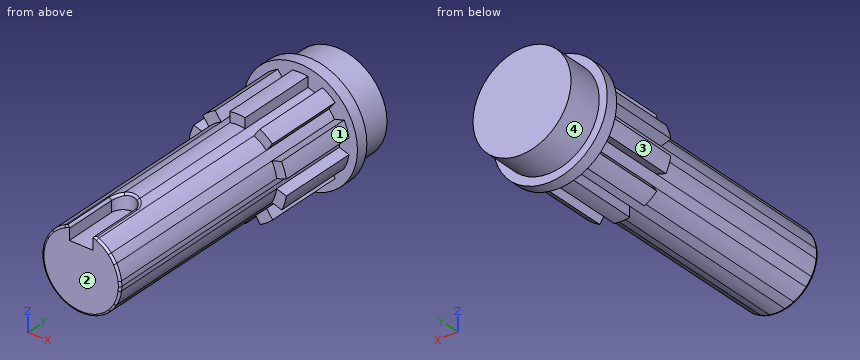
from build123d import *

# Parameters (mm, degrees)
F1_R     = 14.5
F1_R_2   = 12.45
F2_DEPTH = 3
F3_DEPTH = 12
F4_DEPTH = 20
F5_DEPTH = 70
F8_DEPTH = 25
F9_R     = 0.5


with BuildPart() as f2:
    # F1 (on Front) → F2 (new body)
    with BuildSketch(Plane.XZ):
        Circle(F1_R)
        Circle(F1_R_2, mode=Mode.SUBTRACT)
    extrude(amount=-F2_DEPTH)

    # F1 (on Front) → F3 (join)
    with BuildSketch(Plane.XZ):
        Circle(F1_R_2)
    extrude(amount=-F3_DEPTH)

    # F0 (on Front) → F4 (join)
    with BuildSketch(Plane.XZ):
        with BuildLine():
            ThreePointArc((-7.324554284, 6.7344936366), (-5.8782605878, 8.0279855793), (-4.2084272228, 9.0161876816))
            Line((-4.2084272228, 9.0161876816), (-5.7294038305, 11.1096323858))
            ThreePointArc((-5.7294038305, 11.1096323858), (-7.3861439392, 10.0843878203), (-8.8634461682, 8.8141546403))
            Line((-8.8634461682, 8.8141546403), (-7.324554284, 6.7344936366))
        make_face()
        with BuildLine():
            ThreePointArc((-1.9672528507, 9.7535847882), (-0.0368811837, 9.9499316469), (1.8948930083, 9.7679005158))
            Line((1.8948930083, 9.7679005158), (1.8948930083, 12.3555404773))
            ThreePointArc((1.8948930083, 12.3555404773), (-0.0480615306, 12.4999076032), (-1.9898484698, 12.3406038372))
            Line((-1.9898484698, 12.3406038372), (-1.9672528507, 9.7535847882))
        make_face()
        with BuildLine():
            ThreePointArc((4.141472307, 9.047138063), (5.818585579, 8.0713420111), (7.2744285153, 6.7886073517))
            Line((7.2744285153, 6.7886073517), (8.7954051229, 8.8820520559))
            ThreePointArc((8.7954051229, 8.8820520559), (7.3083787492, 10.140887538), (5.6438037116, 11.15336181))
            Line((5.6438037116, 11.15336181), (4.141472307, 9.047138063))
        make_face()
        with BuildLine():
            ThreePointArc((8.668295807, 4.8849920985), (9.4515504169, 3.1097740619), (9.8753795782, 1.2162969155))
            Line((9.8753795782, 1.2162969155), (12.3363714254, 2.015921639))
            ThreePointArc((12.3363714254, 2.015921639), (11.8732667494, 3.9083931094), (11.121714701, 5.7059146602))
            Line((11.121714701, 5.7059146602), (8.668295807, 4.8849920985))
        make_face()
        with BuildLine():
            Line((12.3515086878, -1.9209979529), (9.8841249332, -1.1430548127))
            ThreePointArc((9.8841249332, -1.1430548127), (9.474344242, -3.0396218816), (8.704271294, -4.820597602))
            Line((8.704271294, -4.820597602), (11.1652631412, -5.6202223254))
            ThreePointArc((11.1652631412, -5.6202223254), (11.9029704089, -3.8169746457), (12.3515086878, -1.9209979529))
        make_face()
        with BuildLine():
            Line((8.8634461682, -8.8141546403), (7.324554284, -6.7344936366))
            ThreePointArc((7.324554284, -6.7344936366), (5.8782605878, -8.0279855793), (4.2084272228, -9.0161876816))
            Line((4.2084272228, -9.0161876816), (5.7294038305, -11.1096323858))
            ThreePointArc((5.7294038305, -11.1096323858), (7.3861439392, -10.0843878203), (8.8634461682, -8.8141546403))
        make_face()
        with BuildLine():
            Line((1.9898484698, -12.3406038372), (1.9672528507, -9.7535847882))
            ThreePointArc((1.9672528507, -9.7535847882), (0.0368811837, -9.9499316469), (-1.8948930083, -9.7679005158))
            Line((-1.8948930083, -9.7679005158), (-1.8948930083, -12.3555404773))
            ThreePointArc((-1.8948930083, -12.3555404773), (0.0480615306, -12.4999076032), (1.9898484698, -12.3406038372))
        make_face()
        with BuildLine():
            Line((-5.6438037116, -11.15336181), (-4.141472307, -9.047138063))
            ThreePointArc((-4.141472307, -9.047138063), (-5.818585579, -8.0713420111), (-7.2744285153, -6.7886073517))
            Line((-7.2744285153, -6.7886073517), (-8.7954051229, -8.8820520559))
            ThreePointArc((-8.7954051229, -8.8820520559), (-7.3083787492, -10.140887538), (-5.6438037116, -11.15336181))
        make_face()
        with BuildLine():
            Line((-11.121714701, -5.7059146602), (-8.668295807, -4.8849920985))
            ThreePointArc((-8.668295807, -4.8849920985), (-9.4515504169, -3.1097740619), (-9.8753795782, -1.2162969155))
            Line((-9.8753795782, -1.2162969155), (-12.3363714254, -2.015921639))
            ThreePointArc((-12.3363714254, -2.015921639), (-11.8732667494, -3.9083931094), (-11.121714701, -5.7059146602))
        make_face()
        with BuildLine():
            ThreePointArc((-9.8841249332, 1.1430548127), (-9.474344242, 3.0396218816), (-8.704271294, 4.820597602))
            Line((-8.704271294, 4.820597602), (-11.1652631412, 5.6202223254))
            ThreePointArc((-11.1652631412, 5.6202223254), (-11.9029704089, 3.8169746457), (-12.3515086878, 1.9209979529))
            Line((-12.3515086878, 1.9209979529), (-9.8841249332, 1.1430548127))
        make_face()
    extrude(amount=F4_DEPTH)

    # F0 (on Front) → F5 (join)
    with BuildSketch(Plane.XZ):
        with BuildLine():
            ThreePointArc((9.8841249332, -1.1430548127), (9.9335175815, -0.5724757264), (9.95, 0))
            ThreePointArc((9.95, 0), (9.9313273736, 0.6092918829), (9.8753795782, 1.2162969155))
            ThreePointArc((9.8753795782, 1.2162969155), (9.4515504169, 3.1097740619), (8.668295807, 4.8849920985))
            ThreePointArc((8.668295807, 4.8849920985), (8.0279855793, 5.8782605878), (7.2744285153, 6.7886073517))
            ThreePointArc((7.2744285153, 6.7886073517), (5.818585579, 8.0713420111), (4.141472307, 9.047138063))
            ThreePointArc((4.141472307, 9.047138063), (3.0396218816, 9.474344242), (1.8948930083, 9.7679005158))
            ThreePointArc((1.8948930083, 9.7679005158), (-0.0368811837, 9.9499316469), (-1.9672528507, 9.7535847882))
            ThreePointArc((-1.9672528507, 9.7535847882), (-3.1097740619, 9.4515504169), (-4.2084272228, 9.0161876816))
            ThreePointArc((-4.2084272228, 9.0161876816), (-5.8782605878, 8.0279855793), (-7.324554284, 6.7344936366))
            ThreePointArc((-7.324554284, 6.7344936366), (-8.0713420111, 5.818585579), (-8.704271294, 4.820597602))
            ThreePointArc((-8.704271294, 4.820597602), (-9.474344242, 3.0396218816), (-9.8841249332, 1.1430548127))
            ThreePointArc((-9.8841249332, 1.1430548127), (-9.9499316469, -0.0368811837), (-9.8753795782, -1.2162969155))
            ThreePointArc((-9.8753795782, -1.2162969155), (-9.4515504169, -3.1097740619), (-8.668295807, -4.8849920985))
            ThreePointArc((-8.668295807, -4.8849920985), (-8.0279855793, -5.8782605878), (-7.2744285153, -6.7886073517))
            ThreePointArc((-7.2744285153, -6.7886073517), (-5.818585579, -8.0713420111), (-4.141472307, -9.047138063))
            ThreePointArc((-4.141472307, -9.047138063), (-3.0396218816, -9.474344242), (-1.8948930083, -9.7679005158))
            ThreePointArc((-1.8948930083, -9.7679005158), (0.0368811837, -9.9499316469), (1.9672528507, -9.7535847882))
            ThreePointArc((1.9672528507, -9.7535847882), (3.1097740619, -9.4515504169), (4.2084272228, -9.0161876816))
            ThreePointArc((4.2084272228, -9.0161876816), (5.8782605878, -8.0279855793), (7.324554284, -6.7344936366))
            ThreePointArc((7.324554284, -6.7344936366), (8.0713420111, -5.818585579), (8.704271294, -4.820597602))
            ThreePointArc((8.704271294, -4.820597602), (9.474344242, -3.0396218816), (9.8841249332, -1.1430548127))
        make_face()
    extrude(amount=F5_DEPTH)

    # F7 (on offset) → F8 (cut)
    with BuildSketch(Plane.XY.offset(6)):
        with BuildLine():
            Line((-3, -74.6025964618), (0, -74.6025964618))
            Line((0, -74.6025964618), (3, -74.6025964618))
            Line((3, -74.6025964618), (3, -56.6025964618))
            ThreePointArc((3, -56.6025964618), (0, -53.6025964618), (-3, -56.6025964618))
            Line((-3, -56.6025964618), (-3, -74.6025964618))
        make_face()
    extrude(amount=F8_DEPTH, mode=Mode.SUBTRACT)

    # F9
    f9_edges = [f2.edges().sort_by_distance(p)[0] for p in [
        (-3, -63.301298, 9.486965),
        (0, -53.602596, 9.95),
        (3, -63.301298, 9.486965),
        (-5.377611, -70, -8.371607),
        (7.65146, -70, 6.360634),
    ]]
    fillet(f9_edges, radius=F9_R)


solid = f2.part
Geometry check sheet. Reference: the model listing, model coordinates, mm. Face numbers are marked on the shaded views. A direction names the side the tool comes from. Coordinates: 2 decimals unless noted, no trailing zeros. Use a Markdown table: item, result. Add a question column.
1. Go/stop test with flat-tipped pins: pin 1 Ø6 at (x, y) = (0.5, -34) entering from +Z; pin 2 Ø4 at (x, y) = (-3.5, -20) entering from +Z; pin 3 Ø2 at (x, z) = (-0.5, -10.5) entering from -Y. Record where each tip stops, or that it passes through.
2. Material ranges on L1, parallel to Y at x = -8.5, z = 8.5; L2, parallel to X at y = -19, z = -11.5; L3, parallel to Y at x = 4.5, z = -10.25, recorded low to high.
3. Set-up check for the marked faces 1, 2, 3 and 4: record each of +Z, -Z, +X, -X, +Y, -Y from which the full face is reachable in a straight line by a thin tool's end or side.
Filled sheet:
| question | item | result |
|---|---|---|
| 1 | pin 1 | z = 9.95 |
| 1 | pin 2 | z = 12.41 |
| 1 | pin 3 | y = -70 |
| 2 | L1 | -20 to 12 |
| 2 | L2 | -1.89 to 1.98 |
| 2 | L3 | 0 to 12 |
| 3 | face 1 | +Z, +X, -Y |
| 3 | face 2 | +Z, -Z, +X, -X, -Y |
| 3 | face 3 | -Z, -X, -Y |
| 3 | face 4 | +Y |
